Verification items for this drawing (mm, ordinates from the low corner). A direction names the side the tool comes from. Round coordinates to 2 decimals unless told otherwise and drop trailing zeros. Order: outer loops, then holes, each group sorted by start corner. A loop starts at its lowest first (then second) coordinate and runs counter-clockwise, first axis right, second up. Notation, with made-up numbers: M 77,56 L 99,56 A26 cw 99,91 Z; hole C 24,0 d1. An arc over 180 degrees is marked long. Return JSON: item names as keys, results as strings. Group by question number.
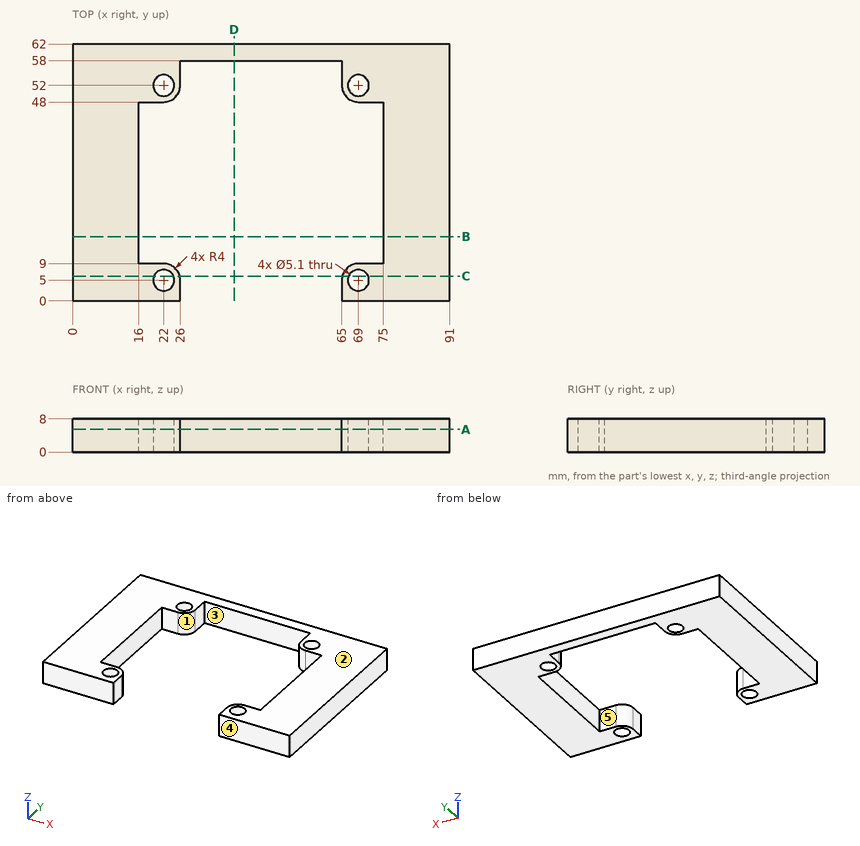
1. Cross-section at A-A (z = 5.5). Enter the section's corners in (x, y).
2. Cross-section at B-B (y = 15.5). Enter the section's corners in (x, z), plus the area to 3 significant figures.
3. Draft check along X on the marked faces 4 and 5. Enter one of: +X half, -X half, draft (parallel to the pull), parting line (faces both ways), or undercut.
4. Go/stop test with flat-tipped pins: pin 1 (4 mm diameter, centred on x = 50.5, z = 4, fed in from -Y); pin 2 (4 mm diameter, centred on x = 17.5, z = 3.5, fed in from -Y). Record where each tip stops, or that it passes through.
5. Thickness scan on line 1 along Y through (x, z) = (69, 4); line 2 along X through (y, z) = (30.5, 1.25); line 3 along X through (y, z) = (55, 6.75). Record the ranges inside material, lowest first. Write a range as from..to.
6. Cross-section at C-C (y = 6). Enter the section's corners in (x, z), plus the area to 3 significant figures.
7. Cross-section at D-D (x = 39). Enter the section's corners in (y, z), plus the area to 3 significant figures.
8. Access from +Z, -Z, +X, -X, +Y, -Y to the whole of each face (thin tool, end or side, straight path). Record for the marked faces 1, 2 and 3.
Computed:
{
 "1": {"outline": "M 0,0 L 26,0 L 26,5 A4 ccw 22,9 L 16,9 L 16,48 L 22,48 A4 ccw 26,52 L 26,58 L 65,58 L 65,52 A4 ccw 69,48 L 75,48 L 75,9 L 69,9 A4 ccw 65,5 L 65,0 L 91,0 L 91,62 L 0,62 Z; hole C 22,5 d5.1; hole C 22,52 d5.1; hole C 69,5 d5.1; hole C 69,52 d5.1"},
 "2": {"outline": "M 0,0 L 16,0 L 16,8 L 0,8 Z; M 75,0 L 91,0 L 91,8 L 75,8 Z", "area": "256 mm²"},
 "3": {"face 4": "draft", "face 5": "undercut"},
 "4": {"pin 1": "stops at y = 58", "pin 2": "stops at y = 0"},
 "5": {"line 1": "y = 0..2.45, 7.55..9, 48..49.45, 54.55..62", "line 2": "x = 0..16, 75..91", "line 3": "x = 0..26, 65..91"},
 "6": {"outline": "M 0,0 L 19.65,0 L 19.65,8 L 0,8 Z; M 24.35,0 L 25.87,0 L 25.87,8 L 24.35,8 Z; M 65.13,0 L 66.65,0 L 66.65,8 L 65.13,8 Z; M 71.35,0 L 91,0 L 91,8 L 71.35,8 Z", "area": "339 mm²"},
 "7": {"outline": "M 58,0 L 62,0 L 62,8 L 58,8 Z", "area": "32.0 mm²"},
 "8": {"face 1": "+Z, -Z", "face 2": "+Z, +X, -X, +Y, -Y", "face 3": "+Z, -Z, -Y"}
}
